Autodesk Inventor part; units mm, degrees
ref_plane "YZ Plane" through (0, 0, 0) normal (1, 0, 0) x (0, 1, 0)
ref_plane "XZ Plane" through (0, 0, 0) normal (0, 1, 0) x (-1, 0, 0)
ref_plane "XY Plane" through (0, 0, 0) normal (0, 0, 1) x (1, 0, 0)
sketch "Szkic1" plane through (0, 0, 0) normal (0, 0, 1) x (1, 0, 0)
  circle A0 centre (0, 0) radius 8
  dimension "d0" = 16
extrude "Wyciągnięcie proste2" add sketch "Szkic1" along normal blind 1000
sketch "Szkic2" plane through (0, 0, 1000) normal (0, 0, 1) x (1, 0, 0)
  circle A0 centre (0, 0) radius 4
  circle A1 centre (0, 0) radius 8
  dimension "d7" = 8
extrude "Wyciągnięcie proste3" cut sketch "Szkic2" against normal blind 30
sketch "Szkic3" plane through (0, 0, 970) normal (0, 0, 1) x (1, 0, 0)
  circle A0 centre (0, 0) radius 8
  circle A1 centre (0, 0) radius 5
  dimension "d10" = 10
extrude "Wyciągnięcie proste4" cut sketch "Szkic3" against normal blind 30
sketch "Szkic4" plane through (0, 0, 970) normal (0, 0, 1) x (1, 0, 0)
  circle A0 centre (0, 0) radius 5
  circle A1 centre (0, 0) radius 4.98
  dimension "d13" = 9.96
extrude "Wyciągnięcie proste5" cut sketch "Szkic4" against normal blind 27
sketch "Szkic5" plane through (0, 0, 0) normal (0, 0, -1) x (-1, 0, 0)
  circle A0 centre (0, 0) radius 5
  circle A1 centre (0, 0) radius 8
  dimension "d18" = 10
extrude "Wyciągnięcie proste6" cut sketch "Szkic5" against normal blind 20
thread "Gwint3"
sketch "Szkic6" plane through (0, 0, 20) normal (0, 0, -1) x (-1, 0, 0)
  circle A0 centre (0, 0) radius 5
  circle A1 centre (0, 0) radius 8
extrude "Wyciągnięcie proste7" cut sketch "Szkic6" against normal blind 329
sketch "Szkic7" plane through (0, 0, 0) normal (0, 0, -1) x (-1, 0, 0)
  circle A0 centre (0, 0) radius 5
extrude "Wyciągnięcie proste8" cut sketch "Szkic7" against normal blind 334
sketch "Szkic8" plane through (0, 0, 940) normal (0, 0, 1) x (1, 0, 0)
  circle A0 centre (0, 0) radius 5
  circle A1 centre (0, 0) radius 8
extrude "Wyciągnięcie proste9" cut sketch "Szkic8" against normal blind 6
sketch "Szkic9" plane through (0, 0, 970) normal (0, 0, 1) x (1, 0, 0)
  circle A0 centre (0, 0) radius 4.98
  circle A1 centre (0, 0) radius 4
extrude "Wyciągnięcie proste10" cut sketch "Szkic9" against normal blind 14
thread "Gwint4"
sketch "Szkic10" plane through (0, 0, 1000) normal (0, 0, 1) x (1, 0, 0)
  circle A0 centre (0, 0) radius 4
extrude "Wyciągnięcie proste11" cut sketch "Szkic10" against normal blind 13.9
properties part number "Śruba trapezowa 16x4 - oś X"
The listing builds one solid part. Answer for the finished solid, in the listing's coordinates (mm). A direction names the side the tool comes from. Coordinates: 2 decimals unless noted, no trailing zeros. Order: outer loops, then holes, each group sorted by start corner. A loop starts at its lowest first (then second) coordinate and runs counter-clockwise, first axis right, second up. Notation, with made-up numbers: M -12.5,-4 L 40.5,-4 A25 cw 40.5,27 Z; hole C 62,-24 d8. An arc over 180 degrees is marked long. Answer as a JSON object with one key per item and string values. Group by question number.
1. A tool of negligible diameter and unlimited length cuts with its end or side. For faces 1 (the cylindrical face through (-1.08, -4.88, 938.56)), 2 (the flat face through (0, 0, 334)), 3 (the flat face through (0.1, -5.2, 349)), from which of +Z, -Z, +X, -X, +Y, -Y can it reach the whole face along a straight path? Write none if from no direction.
2. Straight lines are drawn through the part: line 1 (Z direction, x = 4.75, y = -1.25); line 2 (Z direction, x = 2.5, y = -7); line 3 (Y direction, x = 0.5, z = 914). For each, find the intervals that lie inside material, in ascending order.
3. Section C-C on z = 748.5 is taken. Write down the section's boundary in (x, y).
4. Flat-ended cylindrical pins translate along their axes: P1, Ø1.5, axis at y = -1, z = 687.5, coming from the +X side; P2, Ø1.5, axis at y = 2.5, z = 921, coming from the +X side; P3, Ø6, axis at x = -5, z = 772.5, coming from the -Y side. Find the tip coordinate at first contact, or state that the pin passes through.
Values follow:
{
 "1": {"face 1": "+Z", "face 2": "-Z, +X, -X, +Y, -Y", "face 3": "-Z"},
 "2": {"line 1": "334 to 956", "line 2": "349 to 934", "line 3": "-7.98 to 7.98"},
 "3": {"outline": "C 0,0 d16"},
 "4": {"P1": "x = 8", "P2": "x = 7.81", "P3": "y = -7.75"}
}
